from build123d import *

# Parameters (mm, degrees)
PAD003_DEPTH    = 14.5
SKETCH021_R     = 1.5
POCKET002_DEPTH = 7.25
SKETCH023_W     = 34
SKETCH023_H     = 5
POCKET003_DEPTH = 12.3
CHAMFER006_SIZE = 1
CHAMFER007_SIZE = 1


with BuildPart() as part:
    # Sketch022 → Pad003 (new body)
    with BuildSketch(Plane(origin=(0, 0, 11.5), x_dir=(0, -1, 0), z_dir=(0, 0, 1))):
        Polygon((-15, -23.23103), (15, -23.23103), (17, -9.88), (15, 2), (-15, 2), (-17, -9.88), align=None)
    extrude(amount=PAD003_DEPTH)

    # Sketch021 (on Face8 of Pad003) → Pocket002 (cut)
    with BuildSketch(Plane(origin=(0, 0, 26), x_dir=(0, -1, 0), z_dir=(0, 0, 1))):
        with Locations((11.75, -2.18)):
            Circle(SKETCH021_R)
        with Locations((-11.75, -2.18)):
            Circle(SKETCH021_R)
    extrude(amount=-POCKET002_DEPTH, mode=Mode.SUBTRACT)

    # Sketch023 (on Face8 of Pocket002) → Pocket003 (cut)
    with BuildSketch(Plane(origin=(-23.23103, 0, 11.5), x_dir=(0, -1, 0), z_dir=(-1, 0, 0))):
        with Locations((0, 6.5)):
            Rectangle(SKETCH023_W, SKETCH023_H)
    extrude(amount=-POCKET003_DEPTH, mode=Mode.SUBTRACT)

    # Chamfer006
    chamfer006_edges = [part.edges().sort_by_distance(p)[0] for p in [
        (-10.93103, -16.842554, 18),
        (-10.93103, 16.842554, 18),
    ]]
    chamfer(chamfer006_edges, length=CHAMFER006_SIZE)

    # Chamfer007
    chamfer007_edges = [part.edges().sort_by_distance(p)[0] for p in [
        (-2.18, -10.25, 26),
        (-2.18, 13.25, 26),
    ]]
    chamfer(chamfer007_edges, length=CHAMFER007_SIZE)


solid = part.part
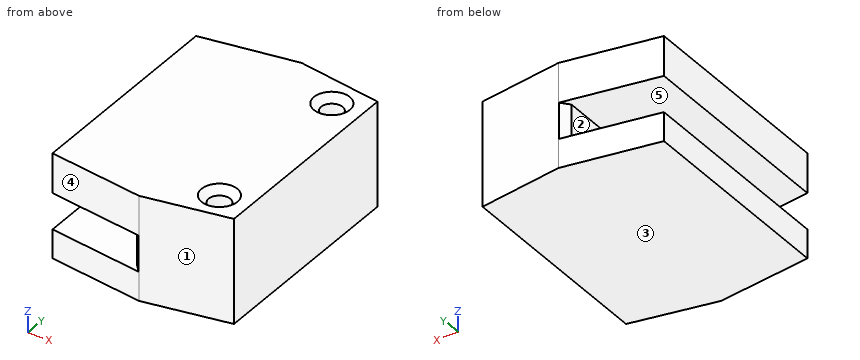
The model under review builds one solid part; all positions refer to its coordinate system, in mm. Face numbers are marked on the shaded views. A direction names the side the tool comes from. Round coordinates to 2 decimals unless told otherwise and drop trailing zeros. Order: outer loops, then holes, each group sorted by start corner. A loop starts at its lowest first (then second) coordinate and runs counter-clockwise, first axis right, second up. Notation, with made-up numbers: (85.5, 52) -> (114.5, 52) arc R23 ccw to (114.5, 78) -> close; hole circle Ø10 at (63.5, 32). An arc over 180 degrees is marked (long way). Write item = value, one per line. Start each with the question number.
Item 1: Consider section C-C on x = -20.25. Write out the cut boundary in (y, z), plus the area to 3 significant figures.
Item 2: Consider section D-D on y = -5.5. Write out the cut boundary in (x, z).
Item 3: Clearance check with flat-ended pins moving along their axes: pin 1 Ø5.5 at (y, z) = (4, 19) entering from -X; pin 2 Ø1.5 at (x, y) = (-2, -12) entering from +Z; pin 3 Ø6 at (x, z) = (-15.5, 16.5) entering from -Y. State where each tip first meets the part, or that it passes through.
Item 4: Mouldability with a two-part tool opening along Z and no side actions: class the marked faces 3, 4 and 5 as released by +Z, released by -Z, zero draft, split by the parting line, or undercut.
Item 5: For line 1 along Z through (x, y) = (-19.25, -3.5); line 2 along X through (y, z) = (11.75, 23); line 3 along X through (y, z) = (14, 17), list the stretches that pass through material, from the lowest coordinate up.
Item 6: Consider section A-A on z = 23.75. Write out the cut boundary in (x, y), plus the area to 3 significant figures.
Item 7: Consider section B-B on y = -11.75. Write out the cut boundary in (x, z), plus the area to 3 significant figures.
Item 8: For the marked faces 1 and 2, list the 3-axis set-ups (+Z, -Z, +X, -X, +Y, -Y) from which the entire face can be reached by the end or side of a thin tool; tool diameter is ignored.
Conclusion:
q1.outline = (-15.45, 11.5) -> (15.45, 11.5) -> (15.45, 15.5) -> (-15.45, 15.5) -> close; (-15.45, 20.5) -> (15.45, 20.5) -> (15.45, 26) -> (-15.45, 26) -> close
q1.area = 293 mm2
q2.outline = (-23.23, 11.5) -> (2, 11.5) -> (2, 26) -> (-23.23, 26) -> (-23.23, 20.5) -> (-10.93, 20.5) -> (-10.93, 15.5) -> (-23.23, 15.5) -> close
q3.pin_1 = -23.23
q3.pin_2 = 18.75
q3.pin_3 = -16.58
q4.face_3 = released by -Z
q4.face_4 = zero draft
q4.face_5 = undercut
q5.line_1 = 11.5 to 15.5, 20.5 to 26
q5.line_2 = -23.23 to -3.68, -0.68 to 2
q5.line_3 = -10.93 to 2
q6.outline = (-23.23, -15) -> (-9.88, -17) -> (2, -15) -> (2, 15) -> (-9.88, 17) -> (-23.23, 15) -> close; hole circle Ø3 at (-2.18, -11.75); hole circle Ø3 at (-2.18, 11.75)
q6.area = 793 mm2
q7.outline = (-23.23, 11.5) -> (2, 11.5) -> (2, 26) -> (0.32, 26) -> (-0.68, 25) -> (-0.68, 18.75) -> (-3.68, 18.75) -> (-3.68, 25) -> (-4.68, 26) -> (-23.23, 26) -> (-23.23, 20.5) -> (-10.93, 20.5) -> (-10.93, 15.5) -> (-23.23, 15.5) -> close
q7.area = 282 mm2
q8.face_1 = +Z, -Z, +X, -Y
q8.face_2 = -X, +Y, -Y
